Geometry check sheet. Reference: the model listing, model coordinates, mm. A direction names the side the tool comes from. Coordinates: 2 decimals unless noted, no trailing zeros. Write each loop counter-clockwise with the first axis right and the second up, starting at its lowest first coordinate (ties: lowest second). Pieces come first, ordered by that corner, then holes. Notation, with made-up numbers: (7.5, 10.5) - (54.5, 10.5) arc R19 ccw to (54.5, 22.5) - close; hole circle Ø1 at (59, 61). An arc over 180 degrees is marked (long way). Answer as a JSON object with one key per item and string values. Group by question number.
from build123d import *

# Parameters (mm, degrees)
SKETCH1_R           = 7
BOSS_EXTRUDE1_DEPTH = 11
SKETCH2_R           = 9.433087352
SKETCH2_R_2         = 7
BOSS_EXTRUDE2_DEPTH = 2


with BuildPart() as part:
    # Sketch1 → Boss-Extrude1 (new body)
    with BuildSketch(Plane(origin=(0, 0, 0), x_dir=(1, 0, 0), z_dir=(0, 1, 0))):
        Circle(SKETCH1_R)
        with BuildLine():
            Line((-6.077951386, 0.85), (-4.977951386, 0.85))
            ThreePointArc((-4.977951386, 0.85), (0, 5.05), (4.977951386, 0.85))
            Line((4.977951386, 0.85), (6.077951386, 0.85))
            Line((6.077951386, 0.85), (6.077951386, -0.85))
            Line((6.077951386, -0.85), (4.977951386, -0.85))
            ThreePointArc((4.977951386, -0.85), (0, -5.05), (-4.977951386, -0.85))
            Line((-4.977951386, -0.85), (-6.077951386, -0.85))
            Line((-6.077951386, -0.85), (-6.077951386, 0.85))
        make_face(mode=Mode.SUBTRACT)
    extrude(amount=BOSS_EXTRUDE1_DEPTH)

    # Sketch2 → Boss-Extrude2 (add)
    with BuildSketch(Plane(origin=(0, 11, 0), x_dir=(1, 0, 0), z_dir=(0, 1, 0))):
        Circle(SKETCH2_R)
        Circle(SKETCH2_R_2, mode=Mode.SUBTRACT)
    extrude(amount=-BOSS_EXTRUDE2_DEPTH)


solid = part.part
(1) Section check B-B (y = 2.5). Record the cut outline in (x, z).
(2) Draft check along X on faces 1 (the face through (9, 10.01, -2.83)), 2 (the face through (-5.5, 5.4, 0.85)), 3 (the face through (5, 0, -2)). Enter one of: +X half, -X half, draft (parallel to the pull), parting line (faces both ways), or undercut.
(3) Section check A-A (z = 0). Record the cut outline in (x, y), and give its area (3 significant figures).
(4) Section check C-C (x = 0). Record the cut outline in (y, z), and give its area (3 significant figures).
(5) Set-up check for faces 4 (the face through (4, 11, 4)), 5 (the face through (6.078, 5, 0)), 6 (the face through (6.466, 4.437, 2.681)): record each of +Z, -Z, +X, -X, +Y, -Y from which the full face is reachable in a straight line by a thin tool's end or side.
(6) Gauge pin test, flat ends, axial feed: pin 1 (1.5 mm diameter, centred on x = -6.5, y = 1, fed in from +Z); pin 2 (2 mm diameter, centred on y = 1.5, z = 2.5, fed in from -X); pin 3 (0.5 mm diameter, centred on y = 5.5, z = -0.5, fed in from -X). Record the tip position at first contact, or that the pin passes through.
(7) Material ranges on L1, parallel to X at y = 4, z = 0; L2, parallel to Y at x = 7, z = -5.25; L3, parallel to Z at x = 5.5, y = 5.25, recorded low to high. Write a range as [from, to].
(8) Section check D-D (z = 8.25). Record the cut outline in (x, y), and give its area (3 significant figures).
Conclusion:
{
 "1": {"outline": "circle Ø14 at (0, 0); hole (-6.08, -0.85) - (-4.98, -0.85) arc R5.05 ccw to (4.98, -0.85) - (6.08, -0.85) - (6.08, 0.85) - (4.98, 0.85) arc R5.05 ccw to (-4.98, 0.85) - (-6.08, 0.85) - close"},
 "2": {"face 1": "parting line", "face 2": "undercut", "face 3": "draft"},
 "3": {"outline": "(-9.43, 9) - (-7, 9) - (-7, 0) - (-6.08, 0) - (-6.08, 11) - (-9.43, 11) - close; (6.08, 0) - (7, 0) - (7, 9) - (9.43, 9) - (9.43, 11) - (6.08, 11) - close", "area": "30.0 mm^2"},
 "4": {"outline": "(0, -7) - (9, -7) - (9, -9.43) - (11, -9.43) - (11, -5.05) - (0, -5.05) - close; (0, 5.05) - (11, 5.05) - (11, 9.43) - (9, 9.43) - (9, 7) - (0, 7) - close", "area": "52.6 mm^2"},
 "5": {"face 4": "+Z, -Z, +X, -X, +Y", "face 5": "+Y, -Y", "face 6": "-Y"},
 "6": {"pin 1": "stops at z = 3.99", "pin 2": "stops at x = -6.84", "pin 3": "stops at x = -7"},
 "7": {"L1": "x = [-7, -6.08], [6.08, 7]", "L2": "y = [9, 11]", "L3": "z = [-4.33, -0.85], [0.85, 4.33]"},
 "8": {"outline": "(-4.57, 9) - (4.57, 9) - (4.57, 11) - (-4.57, 11) - close", "area": "18.3 mm^2"}
}
